```python
from build123d import *

# Parameters (mm, degrees)
F0_R      = 650
F1_DEPTH  = 3
F2_R      = 650
F2_R_2    = 630
F3_DEPTH  = 50
F4_W      = 600
F4_H      = 600
F4_R      = 60
F5_DEPTH  = 25
F6_W      = 604
F6_H      = 604
F6_W_2    = 600
F6_H_2    = 600
F7_DEPTH  = 25
F8_W      = 10
F8_H      = 30
F9_DEPTH  = 25
F10_R     = 6
F11_DEPTH = 500


with BuildPart() as f1:
    # F0 (on Top) → F1 (new body)
    with BuildSketch(Plane.XY):
        Circle(F0_R)
    extrude(amount=F1_DEPTH)

    # F2 (on face) → F3 (join)
    with BuildSketch(Plane.XY.offset(3)):
        Circle(F2_R)
        Circle(F2_R_2, mode=Mode.SUBTRACT)
    extrude(amount=F3_DEPTH)

    # F4 (on face) → F5 (cut)
    with BuildSketch(Plane(origin=(0, 0, 0), x_dir=(1, 0, 0), z_dir=(0, 0, -1))):
        Rectangle(F4_W, F4_H)
        with Locations((468.2388901711, 110)):
            Circle(F4_R)
        with Locations((468.2388901711, -110)):
            Circle(F4_R)
    extrude(amount=-F5_DEPTH, mode=Mode.SUBTRACT)

    # F6 (on face) → F7 (join)
    with BuildSketch(Plane(origin=(0, 0, 0), x_dir=(1, 0, 0), z_dir=(0, 0, -1))):
        Rectangle(F6_W, F6_H)
        Rectangle(F6_W_2, F6_H_2, mode=Mode.SUBTRACT)
    extrude(amount=F7_DEPTH)

    # F8 (on face) → F9 (join)
    with BuildSketch(Plane(origin=(0, 0, 0), x_dir=(1, 0, 0), z_dir=(0, 0, -1))):
        with Locations((-235, -342)):
            Rectangle(F8_W, F8_H)
        with Locations((-205, -342)):
            Rectangle(F8_W, F8_H)
        with Locations((205, -342)):
            Rectangle(F8_W, F8_H)
        with Locations((235, -342)):
            Rectangle(F8_W, F8_H)
    extrude(amount=F9_DEPTH)

    # F10 (on Right) → F11 (cut, symmetric)
    with BuildSketch(Plane.YZ):
        with Locations((342, -13)):
            Circle(F10_R)
    extrude(amount=F11_DEPTH, both=True, mode=Mode.SUBTRACT)


solid = f1.part
```
Can you work these out from the model? Positions are in its coordinate system, mm. A direction names the side the tool comes from. Coordinates: 2 decimals unless noted, no trailing zeros. Loops run counter-clockwise (first coordinate to the right, second up) from the corner with the lowest first, then second, coordinate; pieces in that order, holes last. Notation, with made-up numbers: M 48.5,78 L 53.5,78 A20 cw 53.5,85 Z; hole C 72,39 d9. An arc over 180 degrees is marked long. Put each result on its own line as item: value. Start each with the question number.
(1) Which directions (+Z, -Z, +X, -X, +Y, -Y) give clear straight access to the entire face, cutting with the end or side of a thin tool? Please do faces 4 (the face through (300, 4, -11)), 5 (the face through (411, 9, 3)).
(2) We'd pull the mould along Y, two halves only. Please class faces 1 (the face through (-136.57, -615.02, 27.65)), 2 (the face through (619.984, 195.242, 26.129)), 3 (the face through (-533, 340, 53)): +Y half, -Y half, draft (parallel to the pull), parting line (faces both ways), or undercut.
(3) Will these pins go through, and if not, where does the flat tip stop? pin 1 Ø8 at (x, z) = (-451.5, 1) entering from +Y; pin 2 Ø8 at (x, z) = (-295.5, -16) entering from +Y; pin 3 Ø11 at (x, z) = (235.5, -17) entering from +Y.
(4) Imagine slicing it at B-B on z = 25. List the corners of the cut face in (x, y) for me, and give its area (3 significant figures).
(5) Imagine slicing it at C-C on y = 110. List the corners of the cut face in (x, z) for me.
(6) Imagine slicing it at D-D on y = -428. List the corners of the cut face in (x, z) for me.
(7) I need wall thicknesses on probe 1 along Y at (x, z) = (-232.5, -15); probe 2 along Y at (x, z) = (0, 36); probe 3 along X at (y, z) = (55.5, -13). Which ranges of each line are inside material? Lowest first, please.
(8) Imagine slicing it at A-A on x = -40. List the corners of the cut face in (y, z) for me.
Worked answers:
1. face 4: +Z, -Z
1. face 5: +Z
2. face 1: undercut
2. face 2: parting line
2. face 3: draft
3. pin 1: stops at y = 471.43
3. pin 2: stops at y = 302
3. pin 3: stops at y = 357
4. outline: C 0,0 d1300; hole C 0,0 d1260
4. area: 80,400 mm2
5. outline: M -640.62,0 L -302,0 L -302,-25 L -300,-25 L -300,3 L -620.32,3 L -620.32,53 L -640.62,53 Z; M 300,-25 L 302,-25 L 302,0 L 408.24,0 L 408.24,3 L 300,3 Z; M 528.24,0 L 640.62,0 L 640.62,53 L 620.32,53 L 620.32,3 L 528.24,3 Z
6. outline: M -489.2,0 L 489.2,0 L 489.2,53 L 462.29,53 L 462.29,3 L -462.29,3 L -462.29,53 L -489.2,53 Z
7. probe 1: y = -302 to -300, 300 to 302, 327 to 336.34, 347.66 to 357
7. probe 2: y = -650 to -630, 630 to 650
7. probe 3: x = -302 to -300, 300 to 302
8. outline: M -648.77,0 L -302,0 L -302,-25 L -300,-25 L -300,3 L -628.73,3 L -628.73,53 L -648.77,53 Z; M 300,-25 L 302,-25 L 302,0 L 648.77,0 L 648.77,53 L 628.73,53 L 628.73,3 L 300,3 Z
